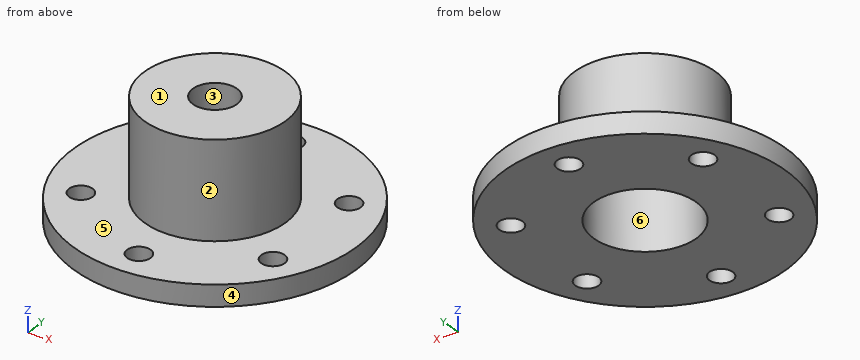
Autodesk Inventor part; units mm, degrees
ref_plane "YZ Plane" through (0, 0, 0) normal (1, 0, 0) x (0, 1, 0)
ref_plane "XZ Plane" through (0, 0, 0) normal (0, 1, 0) x (-1, 0, 0)
ref_plane "XY Plane" through (0, 0, 0) normal (0, 0, 1) x (1, 0, 0)
sketch "Sketch1" plane through (0, 0, 0) normal (0, 0, 1) x (1, 0, 0)
  circle A0 centre (0, 0) radius 30.48
  dimension "d0" = 60.96
extrude "Extrusion1" add sketch "Sketch1" along normal blind 4.572
sketch "Sketch2" plane through (0, 0, 4.572) normal (0, 0, 1) x (1, 0, 0)
  circle A0 centre (0, 0) radius 15.24
  dimension "d3" = 30.48
extrude "Extrusion2" add sketch "Sketch2" along normal blind 20.828
sketch "Sketch3" plane through (0, 0, 25.4) normal (0, 0, 1) x (1, 0, 0)
  circle A0 centre (0, 0) radius 11.1125
  dimension "d6" = 22.225
extrude "Extrusion3" cut sketch "Sketch3" against normal blind 25.4
sketch "Sketch4" plane through (0, 0, 0) normal (0, 0, -1) x (-1, 0, 0)
  circle A0 centre (0, 0) radius 23.8252
  point P0 (0, 23.8252)
  point P1 (-20.6332, 11.9126)
  point P2 (-20.6332, -11.9126)
  point P3 (0, -23.8252)
  point P4 (20.6332, -11.9126)
  point P5 (20.6332, 11.9126)
  dimension "d9" = 23.8252
  dimension "d12" = 360
hole "Hole1" at (0, 23.8252, 0) at (20.6332, 11.9126, 0) at (20.6332, -11.9126, 0) at (0, -23.8252, 0) at (-20.6332, -11.9126, 0) at (-20.6332, 11.9126, 0) direction (0, 0, 1) diameter 5.08 end through all
sketch "Sketch5" plane through (0, 0, 25.4) normal (0, 0, 1) x (1, 0, 0)
  circle A0 centre (0, 0) radius 11.1125
  circle A1 centre (0, 0) radius 4.7625
  dimension "d21" = 9.525
extrude "Extrusion4" add sketch "Sketch5" against normal blind 6.35
properties part number "KHUB"
Could you check a few things on this model? Use its own coordinates, in mm. Face numbers are marked on the shaded views. A direction names the side the tool comes from. Give positions to 0.01 mm unless a question says otherwise; leave off trailing zeros. Loops run counter-clockwise (first coordinate to the right, second up) from the corner with the lowest first, then second, coordinate; pieces in that order, holes last. Notation, with made-up numbers: (57, 25) - (97, 25) arc R27 cw to (97, 59) - close; hole circle Ø10 at (16, 57). An arc over 180 degrees is marked (long way). Use one line per item in the form item = value.
1. I need wall thicknesses on probe 1 along Y at (x, z) = (21.5, 3); probe 2 along Z at (x, y) = (-3, 17); probe 3 along X at (y, z) = (9, 16.5). Which ranges of each line are inside material? Lowest first, please.
Response values:
probe_1 = -21.61 to -14.3, -9.53 to 9.53, 14.3 to 21.61
probe_2 = 0 to 4.57
probe_3 = -12.3 to -6.52, 6.52 to 12.3
2. I want a section at B-B (y = -2.5). Please give me the cut outline in (x, z), and give its area (3 significant figures).
Response values:
outline = (-30.38, 0) - (-10.83, 0) - (-10.83, 19.05) - (-4.05, 19.05) - (-4.05, 25.4) - (-15.03, 25.4) - (-15.03, 4.57) - (-30.38, 4.57) - close; (4.05, 19.05) - (10.83, 19.05) - (10.83, 0) - (30.38, 0) - (30.38, 4.57) - (15.03, 4.57) - (15.03, 25.4) - (4.05, 25.4) - close
area = 440 mm²
3. I'm going to push flat-ended pins straight in: pin 1 Ø4 at (x, z) = (22.5, 4.5) entering from -Y; pin 2 Ø12 at (y, z) = (-8.5, 19) entering from +X; pin 3 Ø6.5 at (x, y) = (-20.63, 11.91) entering from +Z. Where does each tip first touch, or does it pass through?
Response values:
pin_1 = -22.56
pin_2 = 15.03
pin_3 = 4.57
4. I want a section at A-A (x = 0). Please give me the cut outline in (y, z).
Response values:
outline = (-30.48, 0) - (-26.37, 0) - (-26.37, 4.57) - (-30.48, 4.57) - close; (-21.29, 0) - (-11.11, 0) - (-11.11, 19.05) - (-4.76, 19.05) - (-4.76, 25.4) - (-15.24, 25.4) - (-15.24, 4.57) - (-21.29, 4.57) - close; (4.76, 19.05) - (11.11, 19.05) - (11.11, 0) - (21.29, 0) - (21.29, 4.57) - (15.24, 4.57) - (15.24, 25.4) - (4.76, 25.4) - close; (26.37, 0) - (30.48, 0) - (30.48, 4.57) - (26.37, 4.57) - close
5. Thinking about a two-plate mould opening in X: for the marked faces 3, 4, 5 and 6, which applies, released by +X, released by -X, zero draft, split by the parting line, or undercut?
Response values:
face_3 = undercut
face_4 = split by the parting line
face_5 = zero draft
face_6 = undercut
6. I want a section at C-C (z = 3.75). Please give me the cut outline in (x, y) (1 decimal).
Response values:
outline = circle Ø61 at (0, 0); hole circle Ø5.1 at (-20.6, -11.9); hole circle Ø5.1 at (-20.6, 11.9); hole circle Ø22.2 at (0, 0); hole circle Ø5.1 at (0, -23.8); hole circle Ø5.1 at (0, 23.8); hole circle Ø5.1 at (20.6, -11.9); hole circle Ø5.1 at (20.6, 11.9)
7. On a 3-axis mill with a long thin cutter (end or side, diameter ignored), from which of +Z, -Z, +X, -X, +Y, -Y can I reach the whole of each face in a straight line? I mean the marked faces 1 and 2. Say none if no direction works.
Response values:
face_1 = +Z, +X, -X, +Y, -Y
face_2 = +Z
8. I want a section at D-D (z = 14.75). Please give me the cut outline in (x, y) (1 decimal), and give its area (3 significant figures).
Response values:
outline = circle Ø30.5 at (0, 0); hole circle Ø22.2 at (0, 0)
area = 342 mm²
